Source: three-view drawing plus pictorial views. Frame: mm from the lowest corner of the part. Round coordinates to 2 decimals unless told otherwise and drop trailing zeros. Order: outer loops, then holes, each group sorted by start corner. A loop starts at its lowest first (then second) coordinate and runs counter-clockwise, first axis right, second up. Notation, with made-up numbers: M 84.25,85.25 L 134.25,85.25 A26 cw 134.25,101.25 Z; hole C 16.25,-30 d9. An arc over 180 degrees is marked long. Return JSON: item names as keys, results as strings. Group by question number.
Q1. Cut plane B-B on z = 52. Output: boundary loops of the cut face in (x, y), and give its area (3 significant figures).
Q2. Cut plane C-C on y = 0.5. Count the separate pieces of the cut face and the enclosed holes in it, and give its area (3 significant figures).
Q3. Cut plane D-D on z = 32.5. Output: boundary loops of the cut face in (x, y).
Q4. Contact query for a flat-ended pin moving along its axis: pin 1 (1.5 mm diameter, centred on x = 96, z = 20, fed in from -Y). Output: stop coordinate, or through.
Q5. Cut plane A-A on x = 60. Output: boundary loops of the cut face in (y, z), and give its area (4 significant figures).
Q6. Ray query, probe 1 along X at (y, z) = (0.85, 4); probe 2 along Z at (x, y) = (116, 0.5); probe 3 along X at (y, z) = (1.25, 63). Return the intervals inside material, ascending.
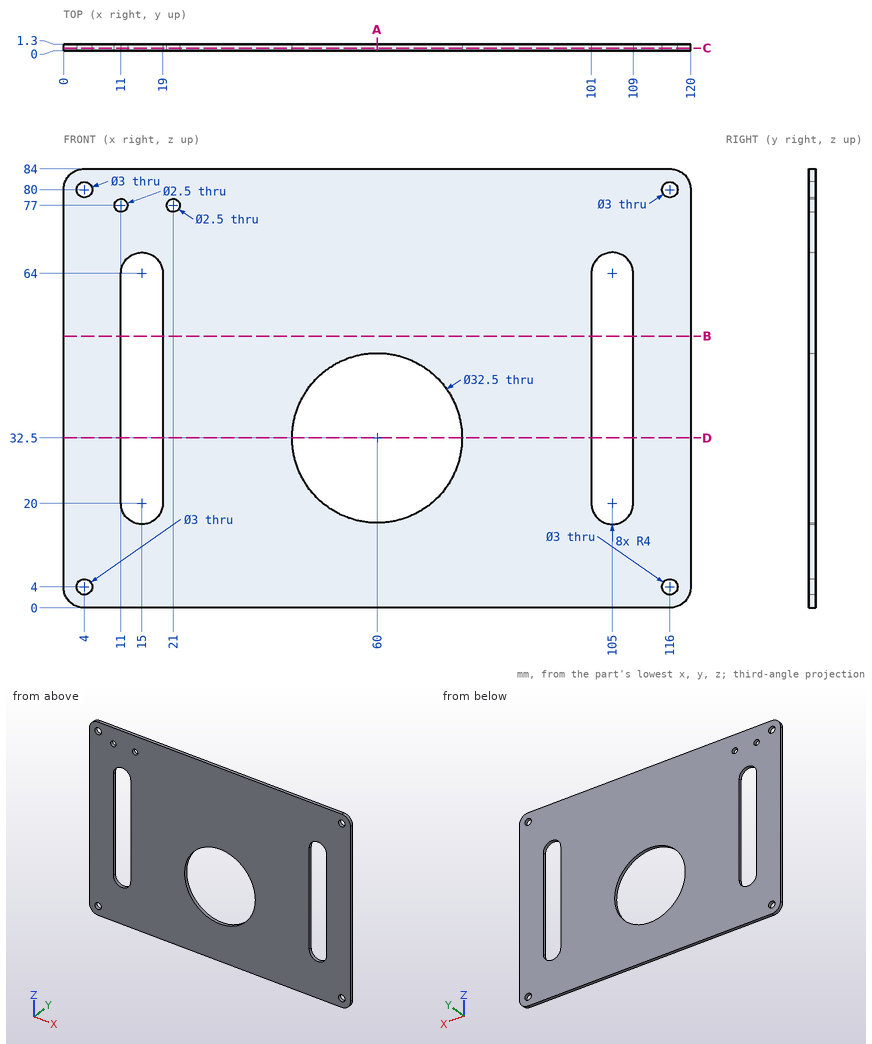
Result sheet:
{
 "1": {"outline": "M 0,0 L 11,0 L 11,1.3 L 0,1.3 Z; M 19,0 L 101,0 L 101,1.3 L 19,1.3 Z; M 109,0 L 120,0 L 120,1.3 L 109,1.3 Z", "area": "135 mm²"},
 "2": {"separate pieces": "1", "enclosed holes": "9", "area": "8,390 mm²"},
 "3": {"outline": "M 0,0 L 11,0 L 11,1.3 L 0,1.3 Z; M 19,0 L 43.75,0 L 43.75,1.3 L 19,1.3 Z; M 76.25,0 L 101,0 L 101,1.3 L 76.25,1.3 Z; M 109,0 L 120,0 L 120,1.3 L 109,1.3 Z"},
 "4": {"pin 1": "stops at y = 0"},
 "5": {"outline": "M 0,0 L 1.3,0 L 1.3,16.25 L 0,16.25 Z; M 0,48.75 L 1.3,48.75 L 1.3,84 L 0,84 Z", "area": "66.95 mm²"},
 "6": {"probe 1": "x = 0 to 2.5, 5.5 to 114.5, 117.5 to 120", "probe 2": "z = 0 to 2.5, 5.5 to 78.5, 81.5 to 84", "probe 3": "x = 0 to 11, 19 to 101, 109 to 120"}
}
